CAD build for the part. Positions are in the model's coordinates, mm. A direction names the side the tool comes from. Give positions to 0.01 mm unless a question says otherwise; leave off trailing zeros. Order: outer loops, then holes, each group sorted by start corner. A loop starts at its lowest first (then second) coordinate and runs counter-clockwise, first axis right, second up. Notation, with made-up numbers: (61.25, 52) -> (68.25, 52) arc R21 ccw to (68.25, 90) -> close; hole circle Ø5 at (7.5, 33). An arc over 180 degrees is marked (long way). Answer as CSV lines item,"result".
Autodesk Inventor part; units mm, degrees
ref_plane "YZ Plane" through (0, 0, 0) normal (1, 0, 0) x (0, 1, 0)
ref_plane "XZ Plane" through (0, 0, 0) normal (0, 1, 0) x (-1, 0, 0)
ref_plane "XY Plane" through (0, 0, 0) normal (0, 0, 1) x (1, 0, 0)
sketch "Sketch1" plane through (0, 0, 0) normal (0, 0, 1) x (1, 0, 0)
  line L0 (-10, -10) -> (-5.6, -10)
  line L1 (-10, -5.6) -> (-10, -10)
  line L2 (-5.6, -10) -> (-5, -10)
  line L3 (-3.2, -8.2) -> (-5.6, -8.2)
  line L4 (-2.8351, -3.825) -> (-5.6, -6.5899)
  line L5 (-3.825, -2.8351) -> (-6.5899, -5.6)
  line L6 (0, 0) -> (0, -11) construction
  line L7 (0, 0) -> (-12, 0) construction
  line L8 (-3.2, -8.2) -> (-5, -10)
  line L9 (-6.5899, -5.6) -> (-8.2, -5.6)
  line L10 (-10, -5.6) -> (-10, -5)
  line L11 (-10, -5) -> (-8.2, -3.2)
  line L12 (-8.2, -3.2) -> (-8.2, -5.6)
  line L13 (-5.6, -8.2) -> (-5.6, -6.5899)
  arc A0 (-2.15, 0) -> (0, -2.15) centre (0, 0) ccw
  line L14 (0, 0) -> (-3.825, 0)
  line L15 (-3.825, 0) -> (-3.825, -2.8351)
  line L16 (-2.8351, -3.825) -> (0, -3.825)
  line L17 (0, -3.825) -> (0, 0)
  line L18 (-2.8351, -3.825) -> (-3.825, -3.825) construction
  line L19 (-3.825, -3.825) -> (-3.825, -2.8351) construction
  line L20 (3.825, -2.8351) -> (3.825, -3.825) construction
  line L21 (3.825, -2.8351) -> (3.825, 0)
  line L22 (3.825, -3.825) -> (2.8351, -3.825) construction
  line L23 (3.825, 0) -> (0, 0)
  line L24 (0, -3.825) -> (2.8351, -3.825)
  arc A1 (0, -2.15) -> (2.15, 0) centre (0, 0) ccw
  line L25 (0, 0) -> (0, -3.825)
  line L26 (2.8351, -3.825) -> (5.6, -6.5899)
  line L27 (0, 0) -> (0, -12) construction
  line L28 (0, 0) -> (11, 0) construction
  line L29 (3.825, -2.8351) -> (6.5899, -5.6)
  line L30 (8.2, -3.2) -> (8.2, -5.6)
  line L31 (10, -5.6) -> (10, -5)
  line L32 (8.2, -3.2) -> (10, -5)
  line L33 (8.2, -5.6) -> (6.5899, -5.6)
  line L34 (5.6, -6.5899) -> (5.6, -8.2)
  line L35 (10, -10) -> (10, -5.6)
  line L36 (5.6, -10) -> (10, -10)
  line L37 (3.2, -8.2) -> (5.6, -8.2)
  line L38 (5, -10) -> (3.2, -8.2)
  line L39 (5.6, -10) -> (5, -10)
  line L40 (2.8351, 3.825) -> (3.825, 3.825) construction
  line L41 (2.8351, 3.825) -> (0, 3.825)
  line L42 (3.825, 3.825) -> (3.825, 2.8351) construction
  line L43 (0, 3.825) -> (0, 0)
  line L44 (3.825, 0) -> (3.825, 2.8351)
  arc A2 (2.15, 0) -> (0, 2.15) centre (0, 0) ccw
  line L45 (0, 0) -> (3.825, 0)
  line L46 (3.825, 2.8351) -> (6.5899, 5.6)
  line L47 (0, 0) -> (12, 0) construction
  line L48 (0, 0) -> (0, 11) construction
  line L49 (2.8351, 3.825) -> (5.6, 6.5899)
  line L50 (3.2, 8.2) -> (5.6, 8.2)
  line L51 (5.6, 10) -> (5, 10)
  line L52 (3.2, 8.2) -> (5, 10)
  line L53 (5.6, 8.2) -> (5.6, 6.5899)
  line L54 (6.5899, 5.6) -> (8.2, 5.6)
  line L55 (10, 10) -> (5.6, 10)
  line L56 (10, 5.6) -> (10, 10)
  line L57 (8.2, 3.2) -> (8.2, 5.6)
  line L58 (10, 5) -> (8.2, 3.2)
  line L59 (10, 5.6) -> (10, 5)
  line L60 (-3.825, 2.8351) -> (-3.825, 3.825) construction
  line L61 (-3.825, 2.8351) -> (-3.825, 0)
  line L62 (-3.825, 3.825) -> (-2.8351, 3.825) construction
  line L63 (-3.825, 0) -> (0, 0)
  line L64 (0, 3.825) -> (-2.8351, 3.825)
  arc A3 (0, 2.15) -> (-2.15, 0) centre (0, 0) ccw
  line L65 (0, 0) -> (0, 3.825)
  line L66 (-2.8351, 3.825) -> (-5.6, 6.5899)
  line L67 (0, 0) -> (0, 12) construction
  line L68 (0, 0) -> (-11, 0) construction
  line L69 (-3.825, 2.8351) -> (-6.5899, 5.6)
  line L70 (-8.2, 3.2) -> (-8.2, 5.6)
  line L71 (-10, 5.6) -> (-10, 5)
  line L72 (-8.2, 3.2) -> (-10, 5)
  line L73 (-8.2, 5.6) -> (-6.5899, 5.6)
  line L74 (-5.6, 6.5899) -> (-5.6, 8.2)
  line L75 (-10, 10) -> (-10, 5.6)
  line L76 (-5.6, 10) -> (-10, 10)
  line L77 (-3.2, 8.2) -> (-5.6, 8.2)
  line L78 (-5, 10) -> (-3.2, 8.2)
  line L79 (-5.6, 10) -> (-5, 10)
  point P0 (0, 2.15)
  point P1 (2.15, 0)
  point P2 (0, -2.15)
  dimension "d16" = 10
  dimension "d19" = 3.2
  dimension "d21" = 4.4
  dimension "d22" = 4.4
  dimension "d24" = 45
  dimension "d25" = 1.8
  dimension "d27" = 1.8
  dimension "d28" = 45
  dimension "d29" = 3.2
  dimension "d31" = 1.4
  dimension "d33" = 2.15
  dimension "d34" = 3.825
  dimension "d35" = 3.825
  dimension "d36" = 135
  dimension "d39" = 360
extrude "Extrusion1" add sketch "Sketch1" along normal blind 70 contours L1 L10 L11 L12 L9 L5 L15 L14 A0 L17 L16 L4 L13 L3 L8 L2 L0 | L17 A1 L23 L21 L29 L33 L30 L32 L31 L35 L36 L39 L38 L37 L34 L26 L24 | L61 L69 L73 L70 L72 L71 L75 L76 L79 L78 L77 L74 L66 L64 L43 A3 L14 | A2 L43 L41 L49 L53 L50 L52 L51 L55 L56 L59 L58 L57 L54 L46 L44 L23
properties part number "AP20x20"
1) Which spindle directions (+Z, -Z, +X, -X, +Y, -Y) get a long thin tool onto all of the face, cutting with end or side? Do faces 1 (the flat face through (-5.6, -7, 35)), 2 (the flat face through (-9, -4, 35)), 3 (the flat face through (-4, 9, 35)), 4 (the flat face through (9, -4, 35)). Say none if no direction does.
Data:
face 1,"+Z, -Z"
face 2,"+Z, -Z, -X"
face 3,"+Z, -Z, +Y"
face 4,"+Z, -Z, +X"
2) Pull direction Z, two halves, no side cores. Call faces 5 (the flat face through (-0.1, 2.4, 0)), 6 (the flat face through (-0.1, 2.4, 70)), 7 (the flat face through (4, 8.2, 35)): pulls with the +Z half, pulls with the -Z half, needs draft (parallel to the pull), parting line crosses it, or undercut.
Data:
face 5,"pulls with the -Z half"
face 6,"pulls with the +Z half"
face 7,"needs draft"
3) Pin check, flat tips, straight feed: P1, Ø0.7, axis at x = 4, z = 32, coming from the -Y side; P2, Ø4, axis at x = -2, z = 7, coming from the -Y side; P3, Ø1.9, axis at x = -4, z = 34, coming from the +Y side. Stop position of each tip, or through.
Data:
P1,"stops at y = -9.35"
P2,"stops at y = -9"
P3,"stops at y = 9.95"
4) Wall check: line 1 along Y through (x, z) = (0, 50) (3 decimals); line 2 along X through (y, z) = (-7.75, 32.5). Give the ranges that are in metal, low to high. Write a range as [from, to].
Data:
line 1,"y = [-3.825, -2.15], [2.15, 3.825]"
line 2,"x = [-10, -5.6], [5.6, 10]"
5) Band-saw the part on B-B, the plane y = 0. Write the cut outline in (x, z) (3 decimals), then the cut area to 4 significant figures.
Data:
outline,"(-3.825, 0) -> (-2.15, 0) -> (-2.15, 70) -> (-3.825, 70) -> close; (2.15, 0) -> (3.825, 0) -> (3.825, 70) -> (2.15, 70) -> close"
area,"234.5 mm2"
6) Band-saw the part on A-A, the plane x = -7.5. Write the cut outline in (y, z), then the cut area to 3 significant figures.
Data:
outline,"(-10, 0) -> (-5.6, 0) -> (-5.6, 70) -> (-10, 70) -> close; (5.6, 0) -> (10, 0) -> (10, 70) -> (5.6, 70) -> close"
area,"616 mm2"
